Build history of the part. All positions in model axes, mm. A direction names the side the tool comes from. Round coordinates to 2 decimals unless told otherwise and drop trailing zeros. Order: outer loops, then holes, each group sorted by start corner. A loop starts at its lowest first (then second) coordinate and runs counter-clockwise, first axis right, second up. Notation, with made-up numbers: M -27.75,44.25 L 16.25,44.25 A20 cw 16.25,58.25 Z; hole C -29.75,58.5 d9. An arc over 180 degrees is marked long. One line per item, written item: value. Start each with the question number.
Item 1: Probe L1, parallel to Z at x = -14.25, y = -2.5; L2, parallel to Z at x = -0.5, y = 1.25. List the from-to ranges inside material, lowest first.
Item 2: Tool access for faces 4 (the flat face through (-12, 0, -2.9)), 5 (the flat face through (-6, -2, 4)), 6 (the flat face through (1, 4, 6)), 7 (the flat face through (-6, 4, -1)): list every direction of +Z, -Z, +X, -X, +Y, -Y with a clear straight run to the whole face (end or side of a thin tool).
Item 3: Band-saw the part on A-A, the plane y = 14.5. Write the cut outline in (x, z), then the cut area to 3 significant figures.
Item 4: Band-saw the part on D-D, the plane z = 14.5. Write the cut outline in (x, y), then the cut area to 3 significant figures.
Item 5: Two-plate mould, pull along X, no slides. Class faces 1 (the flat face through (-4, 6, -1)), 2 (the flat face through (2.9, 0, 12)), 3 (the flat face through (0, 16, 0)): +X half, -X half, draft (parallel to the pull), parting line (faces both ways), or undercut.
Item 6: Pin check, flat tips, straight feed: pin 1 (1.7 mm diameter, centred on x = 0.5, z = 11, fed in from +Y); pin 2 (6.5 mm diameter, centred on x = -10.5, z = -0.5, fed in from +Y); pin 3 (1.7 mm diameter, centred on y = 11, z = 1, fed in from -X). Stop position of each tip, or through.
Item 7: Band-saw the part on C-C, the plane z = -1.25. Write the cut outline in (x, y), then the cut area to 3 significant figures.
Item 8: Band-saw the part on B-B, the plane x = -9.25. Write the cut outline in (y, z).
```python
from build123d import *

# Parameters (mm, degrees)
SKETCH1_W                       = 8
SKETCH1_H                       = 8
BOSS_EXTRUDE1_DEPTH             = 4
SKETCH3_W                       = 5.8
SKETCH3_H                       = 5.8
BOSS_EXTRUDE2_DEPTH             = 12
SKETCH5_W                       = 5.8
SKETCH5_H                       = 5.8
BOSS_EXTRUDE3_DEPTH             = 12
SKETCH6_W                       = 5.8
SKETCH6_H                       = 5.8
BOSS_EXTRUDE4_DEPTH             = 12
BOSS_EXTRUDE5_REACH             = 21.514
BOSS_EXTRUDE5_DIRECTION_2_DEPTH = 10
SKETCH9_W                       = 8
SKETCH9_H                       = 8
BOSS_EXTRUDE6_DEPTH             = 4.1
SKETCH10_W                      = 8
SKETCH10_H                      = 8
BOSS_EXTRUDE7_DEPTH             = 4.1
SKETCH11_W                      = 8
SKETCH11_H                      = 8
BOSS_EXTRUDE8_DEPTH             = 4.1


with BuildPart() as part:
    # Sketch1 → Boss-Extrude1 (new, symmetric)
    with BuildSketch(Plane(origin=(0, 0, 0), x_dir=(1, 0, 0), z_dir=(0, 1, 0))):
        Rectangle(SKETCH1_W, SKETCH1_H)
    extrude(amount=BOSS_EXTRUDE1_DEPTH, both=True)

    # Sketch3 → Boss-Extrude2 (add)
    with BuildSketch(Plane.XY.offset(4)):
        Rectangle(SKETCH3_W, SKETCH3_H)
    extrude(amount=BOSS_EXTRUDE2_DEPTH)

    # Sketch5 → Boss-Extrude3 (add)
    with BuildSketch(Plane(origin=(0, 4, 0), x_dir=(1, 0, 0), z_dir=(0, 1, 0))):
        Rectangle(SKETCH5_W, SKETCH5_H)
    extrude(amount=BOSS_EXTRUDE3_DEPTH)

    # Sketch6 → Boss-Extrude4 (add)
    with BuildSketch(Plane.ZY.offset(4)):
        Rectangle(SKETCH6_W, SKETCH6_H)
    extrude(amount=BOSS_EXTRUDE4_DEPTH)

    # Sketch8 → Boss-Extrude5 (add, up to next)
    with BuildSketch(Plane(origin=(-7.266666667, 7.266666667, 7.266666667), x_dir=(-0.8164965809277261, -0.4082482904638631, -0.408248290463863), z_dir=(0.5773502691896257, -0.5773502691896258, -0.5773502691896257)), mode=Mode.PRIVATE) as boss_extrude5_sk1:
        Polygon((1.061473671, 3.961473671), (-3.961473671, 1.061473671), (-1.061473671, -3.961473671), (3.961473671, -1.061473671), align=None)
    boss_extrude5_tool1 = extrude(boss_extrude5_sk1.sketch, amount=BOSS_EXTRUDE5_REACH, mode=Mode.PRIVATE) - part.part
    add(boss_extrude5_tool1.solids().sort_by_distance((-7.266667, 7.266667, 7.266667))[0])

    # Sketch8 → Boss-Extrude5 direction 2 (add)
    with BuildSketch(Plane(origin=(-7.266666667, 7.266666667, 7.266666667), x_dir=(-0.8164965809277261, -0.4082482904638631, -0.408248290463863), z_dir=(0.5773502691896257, -0.5773502691896258, -0.5773502691896257))):
        Polygon((1.061473671, 3.961473671), (-3.961473671, 1.061473671), (-1.061473671, -3.961473671), (3.961473671, -1.061473671), align=None)
    extrude(amount=-BOSS_EXTRUDE5_DIRECTION_2_DEPTH)

    # Sketch9 → Boss-Extrude6 (add)
    with BuildSketch(Plane.ZY.offset(4)):
        Rectangle(SKETCH9_W, SKETCH9_H)
    extrude(amount=BOSS_EXTRUDE6_DEPTH)

    # Sketch10 → Boss-Extrude7 (add)
    with BuildSketch(Plane.XY.offset(4)):
        Rectangle(SKETCH10_W, SKETCH10_H)
    extrude(amount=BOSS_EXTRUDE7_DEPTH)

    # Sketch11 → Boss-Extrude8 (add)
    with BuildSketch(Plane(origin=(0, 4, 0), x_dir=(1, 0, 0), z_dir=(0, 1, 0))):
        Rectangle(SKETCH11_W, SKETCH11_H)
    extrude(amount=BOSS_EXTRUDE8_DEPTH)


solid = part.part
```
Output:
1. L1: z = -2.9 to 2.9
1. L2: z = -4 to 16
2. face 4: -Z, -X, +Y, -Y
2. face 5: +Z, -X, -Y
2. face 6: +Z, +X, +Y
2. face 7: -Z, -X, +Y
3. outline: M -14.36,10.26 L -13,8.9 L -8.9,13 L -10.26,14.36 Z; M -2.9,-2.9 L 2.9,-2.9 L 2.9,2.9 L -2.9,2.9 Z
3. area: 44.8 mm²
4. outline: M -13.95,10.67 L -10.4,8.9 L -10.4,14.22 Z; M -2.9,-2.9 L 2.9,-2.9 L 2.9,2.9 L -2.9,2.9 Z
4. area: 43.1 mm²
5. face 1: undercut
5. face 2: +X half
5. face 3: draft
6. pin 1: stops at y = 2.9
6. pin 2: stops at y = 4
6. pin 3: stops at x = -2.9
7. outline: M -16,-2.9 L -8.1,-2.9 L -8.1,-4 L 4,-4 L 4,8.1 L 2.9,8.1 L 2.9,16 L -2.9,16 L -2.9,8.1 L -4,8.1 L -4,4 L -8.1,4 L -8.1,2.9 L -16,2.9 Z
7. area: 221 mm²
8. outline: M -2.9,-2.9 L 2.9,-2.9 L 2.9,2.9 L -2.9,2.9 Z; M 3.65,5.15 L 10.75,5.15 L 14.85,13.35 L 7.75,13.35 Z
